from build123d import *

# Parameters (mm, degrees)
SKETCH1_R           = 4
BOSS_EXTRUDE1_DEPTH = 4.6
SKETCH2_R           = 2.5
BOSS_EXTRUDE2_DEPTH = 69
CHAMFER1_SIZE       = 0.3
CHAMFER2_SIZE       = 0.3


with BuildPart() as part:
    # Sketch1 → Boss-Extrude1 (new body)
    with BuildSketch(Plane(origin=(0, 0, 0), x_dir=(1, 0, 0), z_dir=(0, 1, 0))):
        with Locations(Location((0, 0, 0), (0, 0, 270))):
            Circle(SKETCH1_R)
    extrude(amount=BOSS_EXTRUDE1_DEPTH)

    # Sketch2 → Boss-Extrude2 (add)
    with BuildSketch(Plane(origin=(0, 4.6, 0), x_dir=(1, 0, 0), z_dir=(0, 1, 0))):
        with Locations(Location((0, 0, 0), (0, 0, 270))):
            Circle(SKETCH2_R)
    extrude(amount=BOSS_EXTRUDE2_DEPTH)

    # Chamfer1
    chamfer1_edges = [part.edges().sort_by_distance(p)[0] for p in [
        (0, 0, -4),
        (0, 4.6, -4),
    ]]
    chamfer(chamfer1_edges, length=CHAMFER1_SIZE)

    # Chamfer2
    chamfer2_edges = [part.edges().sort_by_distance(p)[0] for p in [
        (0, 73.6, -2.5),
    ]]
    chamfer(chamfer2_edges, length=CHAMFER2_SIZE)


solid = part.part
Geometry: final body of the model. Coordinates: model frame, mm. A direction names the side the tool comes from. Coordinates: 2 decimals unless noted, no trailing zeros. Loops run counter-clockwise (first coordinate to the right, second up) from the corner with the lowest first, then second, coordinate; pieces in that order, holes last. Notation, with made-up numbers: M 86.5,79 L 126.5,79 A37 ccw 126.5,117 Z; hole C -40,6 d5. An arc over 180 degrees is marked long. One line per item, written item: value. Start each with the question number.
1) Cut plane A-A (x = 0). Return loops of the section in (y, z), then the cut area to 3 significant figures.
2) Pin query (flat end, axial travel): P1, Ø3, axis at y = 27, z = -2.5, coming from the -X side; P2, Ø4, axis at x = 0, y = 22.5, coming from the +Z side; P3, Ø2, axis at x = -1.5, z = 3, coming from the -Y side; P4, Ø1.5, axis at x = 1, y = 59.5, coming from the -Z side. Return the tip coordinate at first contact, or that it passes through.
3) Material intervals for L1, parallel to Y at x = -3.5, z = -0.5; L2, parallel to Z at x = -1.5, y = 63, sorted ascending. Write a range as from..to.
4) Cut plane B-B (z = 0). Return loops of the section in (x, y).
5) Reachability of faces 1 (the flat face through (3, 4.6, 0)), 2 (the flat face through (0, 73.6, 0)) from +Z, -Z, +X, -X, +Y, -Y: full face, straight path, thin tool, end or side. Return the list, or none.
6) Cut plane C-C (y = 25.5). Return loops of the section in (x, z), then the cut area to 3 significant figures.
Evaluation:
1. outline: M 0,-3.7 L 0.3,-4 L 4.3,-4 L 4.6,-3.7 L 4.6,-2.5 L 73.3,-2.5 L 73.6,-2.2 L 73.6,2.2 L 73.3,2.5 L 4.6,2.5 L 4.6,3.7 L 4.3,4 L 0.3,4 L 0,3.7 Z
1. area: 382 mm^2
2. P1: x = -2.29
2. P2: z = 2.5
2. P3: y = 0
2. P4: z = -2.49
3. L1: 0..4.6
3. L2: -2..2
4. outline: M -4,0.3 L -3.7,0 L 3.7,0 L 4,0.3 L 4,4.3 L 3.7,4.6 L 2.5,4.6 L 2.5,73.3 L 2.2,73.6 L -2.2,73.6 L -2.5,73.3 L -2.5,4.6 L -3.7,4.6 L -4,4.3 Z
5. face 1: +Y
5. face 2: +Z, -Z, +X, -X, +Y
6. outline: C 0,0 d5
6. area: 19.6 mm^2
